Read the model definition and answer for the solid it produces. Units are mm, in the model's axes. Face numbers are marked on the shaded views. Round coordinates to 2 decimals unless told otherwise and drop trailing zeros. Loops run counter-clockwise (first coordinate to the right, second up) from the corner with the lowest first, then second, coordinate; pieces in that order, holes last. Notation, with made-up numbers: (63, 55) - (111, 55) arc R19 ccw to (111, 84) - close; hole circle Ø8 at (57.25, 87.5). An arc over 180 degrees is marked (long way). Use one line per item in the form item = value. Start each with the question number.
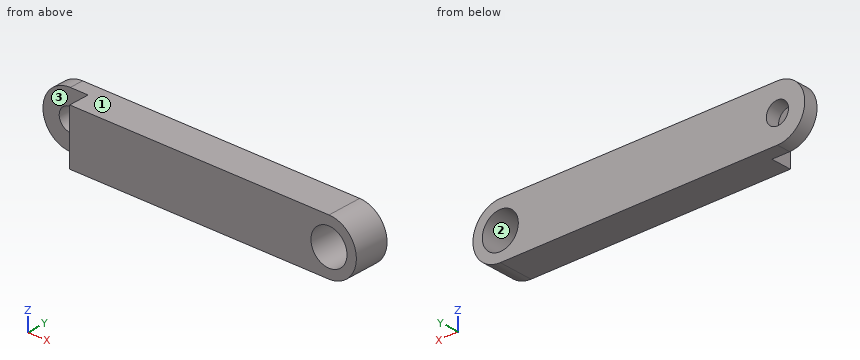
```python
from build123d import *

# Parameters (mm, degrees)
SKETCH1_R           = 1.6
SKETCH1_R_2         = 2.6
BOSS_EXTRUDE1_DEPTH = 5
SKETCH2_R           = 1.6
CUT_EXTRUDE1_DEPTH  = 3


with BuildPart() as part:
    # Sketch1 → Boss-Extrude1 (new body)
    with BuildSketch(Plane(origin=(0, 0, 0), x_dir=(1, 0, 0), z_dir=(0, 1, 0))):
        with BuildLine():
            Line((0, 3.95), (40, 3.95))
            ThreePointArc((40, 3.95), (43.95, 0), (40, -3.95))
            Line((40, -3.95), (0, -3.95))
            ThreePointArc((0, -3.95), (-3.95, 0), (0, 3.95))
        make_face()
        Circle(SKETCH1_R, mode=Mode.SUBTRACT)
        with Locations((40, 0)):
            Circle(SKETCH1_R_2, mode=Mode.SUBTRACT)
    extrude(amount=BOSS_EXTRUDE1_DEPTH)

    # Sketch2 → Cut-Extrude1 (cut)
    with BuildSketch(Plane.XZ):
        with BuildLine():
            Line((2.569533032, 3), (2.569533032, -3))
            Line((2.569533032, -3), (2.569533032, -3.95))
            Line((2.569533032, -3.95), (0, -3.95))
            ThreePointArc((0, -3.95), (-3.95, 0), (0, 3.95))
            Line((0, 3.95), (2.569533032, 3.95))
            Line((2.569533032, 3.95), (2.569533032, 3))
        make_face()
        Circle(SKETCH2_R, mode=Mode.SUBTRACT)
    extrude(amount=-CUT_EXTRUDE1_DEPTH, mode=Mode.SUBTRACT)


solid = part.part
```
1) A cutting plane is placed at A-A on z = 0. Write down the section's boundary in (x, y).
2) A cutting plane is placed at C-C on z = -2. Write down the section's boundary in (x, y), plus the area to 3 significant figures.
3) A cutting plane is placed at D-D on z = 3.5. Write down the section's boundary in (x, y).
4) Determine the mould class of the marked faces 1, 2 and 3 for opening direction Z: +Z half, -Z half, draft (parallel to the pull), parting line (faces both ways), or undercut.
5) A cutting plane is placed at B-B on y = 1.9. Write down the section's boundary in (x, z), plus the area to 3 significant figures.
6) Straight lines are drawn through the part: line 1 (X direction, y = 4.05, z = 0); line 2 (Z direction, x = 40, y = 2.6); line 3 (X direction, y = 2.55, z = 0). For each, find the intervals that lie inside material, in ascending order. Write a range as from..to.
7) Flat-ended cylindrical pins translate along their axes: pin 1 (1.9 mm diameter, centred on x = 0, z = 0, fed in from +Y); pin 2 (1.5 mm diameter, centred on y = 1, z = 0, fed in from -X); pin 3 (2 mm diameter, centred on y = 2.5, z = -2.5, fed in from +X). Find the tip coordinate at first contact, or state that the pin passes through.
Checks:
q1.outline = (-3.95, 3) - (-1.6, 3) - (-1.6, 5) - (-3.95, 5) - close; (1.6, 3) - (2.57, 3) - (2.57, 0) - (37.4, 0) - (37.4, 5) - (1.6, 5) - close; (42.6, 0) - (43.95, 0) - (43.95, 5) - (42.6, 5) - close
q2.outline = (-3.41, 3) - (2.57, 3) - (2.57, 0) - (38.34, 0) - (38.34, 5) - (-3.41, 5) - close; (41.66, 0) - (43.41, 0) - (43.41, 5) - (41.66, 5) - close
q2.area = 200 mm²
q3.outline = (-1.83, 3) - (2.57, 3) - (2.57, 0) - (41.83, 0) - (41.83, 5) - (-1.83, 5) - close
q4.face_1 = +Z half
q4.face_2 = undercut
q4.face_3 = draft
q5.outline = (2.57, -3.95) - (40, -3.95) arc R3.95 ccw to (40, 3.95) - (2.57, 3.95) - close; hole circle Ø5.2 at (40, 0)
q5.area = 299 mm²
q6.line_1 = -3.95..-1.6, 1.6..37.4, 42.6..43.95
q6.line_2 = -3.95..-2.6, 2.6..3.95
q6.line_3 = 2.57..37.4, 42.6..43.95
q7.pin_1 = through
q7.pin_2 = 2.57
q7.pin_3 = 43.65
